Source: CAD feature listing. Evaluate the final solid. Frame: model axes, mm. A direction names the side the tool comes from. Round coordinates to 2 decimals unless told otherwise and drop trailing zeros. Write each loop counter-clockwise with the first axis right and the second up, starting at its lowest first coordinate (ties: lowest second). Pieces come first, ordered by that corner, then holes.
from build123d import *

# Parameters (mm, degrees)
SKETCH1_R           = 3.5
SKETCH1_R_2         = 1.5
BOSS_EXTRUDE1_DEPTH = 8.25
BOSS_EXTRUDE2_START = 2.8
SKETCH2_R           = 6
SKETCH2_R_2         = 3.5
SKETCH2_R_3         = 1.5
BOSS_EXTRUDE2_DEPTH = 2.8
BOSS_EXTRUDE3_START = 4.8
SKETCH2_3_R         = 6
SKETCH2_3_R_2       = 3.5
SKETCH2_3_R_3       = 1.5
BOSS_EXTRUDE3_DEPTH = 2


with BuildPart() as part:
    # Sketch1 → Boss-Extrude1 (new body)
    with BuildSketch(Plane.XY):
        Circle(SKETCH1_R)
        Circle(SKETCH1_R_2, mode=Mode.SUBTRACT)
    extrude(amount=BOSS_EXTRUDE1_DEPTH)

    # Sketch2 → Boss-Extrude2 (add)
    # profile 1 of 4: a face of its own
    with BuildSketch(Plane(origin=(0, 0, 0), x_dir=(-1, 0, 0), z_dir=(0, 0, -1)).offset(BOSS_EXTRUDE2_START)):
        with BuildLine():
            ThreePointArc((5.984674304, 34.571428571), (0, 29), (-5.984674304, 34.571428571))
            Line((-5.984674304, 34.571428571), (-3.491060011, -0.25))
            ThreePointArc((-3.491060011, -0.25), (-0.125079898, 3.497764289), (3.5, 0))
            ThreePointArc((3.5, 0), (3.497764289, -0.125079898), (3.491060011, -0.25))
            Line((3.491060011, -0.25), (5.984674304, 34.571428571))
        make_face()
    # profile 2 of 4: a face of its own
    with BuildSketch(Plane(origin=(0, 0, 0), x_dir=(-1, 0, 0), z_dir=(0, 0, -1)).offset(BOSS_EXTRUDE2_START)):
        with Locations((0, 35)):
            Circle(SKETCH2_R)
        with Locations((0, 35)):
            Circle(SKETCH2_R_2, mode=Mode.SUBTRACT)
    # profile 3 of 4: a face of its own
    with BuildSketch(Plane(origin=(0, 0, 0), x_dir=(-1, 0, 0), z_dir=(0, 0, -1)).offset(BOSS_EXTRUDE2_START)):
        with Locations(Location((0, 0, 0), (0, 0, 355.903956242))):
            Circle(SKETCH2_R_2)
        with Locations(Location((0, 0, 0), (0, 0, 180))):
            Circle(SKETCH2_R_3, mode=Mode.SUBTRACT)
    # profile 4 of 4: a face of its own
    with BuildSketch(Plane(origin=(0, 0, 0), x_dir=(-1, 0, 0), z_dir=(0, 0, -1)).offset(BOSS_EXTRUDE2_START)):
        with Locations(Location((0, 0, 0), (0, 0, 180))):
            Circle(SKETCH2_R_3)
    extrude(amount=-BOSS_EXTRUDE2_DEPTH)

    # Sketch2<3> → Boss-Extrude3 (add)
    # profile 1 of 5: a face of its own
    with BuildSketch(Plane(origin=(0, 0, 0), x_dir=(-1, 0, 0), z_dir=(0, 0, -1)).offset(BOSS_EXTRUDE3_START)):
        with Locations((0, 35)):
            Circle(SKETCH2_3_R)
        with Locations((0, 35)):
            Circle(SKETCH2_3_R_2, mode=Mode.SUBTRACT)
    # profile 2 of 5: a face of its own
    with BuildSketch(Plane(origin=(0, 0, 0), x_dir=(-1, 0, 0), z_dir=(0, 0, -1)).offset(BOSS_EXTRUDE3_START)):
        with BuildLine():
            ThreePointArc((5.984674304, 34.571428571), (0, 29), (-5.984674304, 34.571428571))
            Line((-5.984674304, 34.571428571), (-3.491060011, -0.25))
            ThreePointArc((-3.491060011, -0.25), (-0.125079898, 3.497764289), (3.5, 0))
            ThreePointArc((3.5, 0), (3.497764289, -0.125079898), (3.491060011, -0.25))
            Line((3.491060011, -0.25), (5.984674304, 34.571428571))
        make_face()
    # profile 3 of 5: a face of its own
    with BuildSketch(Plane(origin=(0, 0, 0), x_dir=(-1, 0, 0), z_dir=(0, 0, -1)).offset(BOSS_EXTRUDE3_START)):
        with Locations(Location((0, 0, 0), (0, 0, 355.903956242))):
            Circle(SKETCH2_3_R_2)
        with Locations(Location((0, 0, 0), (0, 0, 180))):
            Circle(SKETCH2_3_R_3, mode=Mode.SUBTRACT)
    # profile 4 of 5: a face of its own
    with BuildSketch(Plane(origin=(0, 0, 0), x_dir=(-1, 0, 0), z_dir=(0, 0, -1)).offset(BOSS_EXTRUDE3_START)):
        with Locations((0, 35)):
            Circle(SKETCH2_3_R_2)
    # profile 5 of 5: a face of its own
    with BuildSketch(Plane(origin=(0, 0, 0), x_dir=(-1, 0, 0), z_dir=(0, 0, -1)).offset(BOSS_EXTRUDE3_START)):
        with Locations(Location((0, 0, 0), (0, 0, 180))):
            Circle(SKETCH2_3_R_3)
    extrude(amount=-BOSS_EXTRUDE3_DEPTH)


solid = part.part
1) Section query C-C on x = 0. Return the cut outline in (y, z), then the cut area to 3 significant figures.
Taken from the geometry:
outline: (-3.5, -4.8) - (41, -4.8) - (41, 0) - (38.5, 0) - (38.5, -2.8) - (31.5, -2.8) - (31.5, 0) - (3.5, 0) - (3.5, 8.25) - (1.5, 8.25) - (1.5, 0) - (-1.5, 0) - (-1.5, 8.25) - (-3.5, 8.25) - close
area: 227 mm2
2) Reachability of faces 1 (the face through (0, -2, 8.25)), 2 (the face through (-1.5, 0.07, 4.07)) from +Z, -Z, +X, -X, +Y, -Y: full face, straight path, thin tool, end or side. Return the list, or none.
Taken from the geometry:
face 1: +Z, +X, -X, +Y, -Y
face 2: +Z
3) Pull-direction query (Y, two-part tool) for faces 3 (the face through (4.755, 17.404, -2.434)), 4 (the face through (0, 19, -4.8)), 5 (the face through (0, 35, -2.8)); classes: released by +Y, released by -Y, zero draft, split by the parting line, or undercut.
Taken from the geometry:
face 3: released by -Y
face 4: zero draft
face 5: undercut
4) Contact query for flat-ended pins moving along their axis: P1, Ø6, axis at x = 1.5, y = 33, coming from the +Z side; P2, Ø3, axis at x = 3, z = 3, coming from the +Y side; P3, Ø4, axis at x = 0, y = 35, coming from the +Z side. Output: stop coordinate, or through.
Taken from the geometry:
P1: stops at z = 0
P2: stops at y = 3.16
P3: stops at z = -2.8
5) Material intervals for line 1 (Y direction, x = 0, z = 6); line 2 (Y direction, x = 0, z = -2.1); line 3 (Z direction, x = -1.5, y = 29.5), sorted ascending.
Taken from the geometry:
line 1: y = -3.5 to -1.5, 1.5 to 3.5
line 2: y = -3.5 to 31.5, 38.5 to 41
line 3: z = -4.8 to 0
6) Section query D-D on x = -2. Return the cut outline in (y, z), then the cut area to 3 significant figures.
Taken from the geometry:
outline: (-2.87, -4.8) - (40.66, -4.8) - (40.66, 0) - (37.87, 0) - (37.87, -2.8) - (32.13, -2.8) - (32.13, 0) - (2.87, 0) - (2.87, 8.25) - (-2.87, 8.25) - close
area: 240 mm2
7) Section query B-B on y = 35. Return the cut outline in (x, z).
Taken from the geometry:
outline: (-6, -4.8) - (6, -4.8) - (6, 0) - (3.5, 0) - (3.5, -2.8) - (-3.5, -2.8) - (-3.5, 0) - (-6, 0) - close
8) Section query A-A on z = -2.25. Return the cut outline in (x, y).
Taken from the geometry:
outline: (-5.98, 34.57) - (-3.49, -0.25) arc R3.5 ccw to (3.49, -0.25) - (5.98, 34.57) arc R6 ccw (long way) to start; hole circle Ø7 at (0, 35)
